Autodesk Inventor part; units mm, degrees
ref_plane "YZ Plane" through (0, 0, 0) normal (1, 0, 0) x (0, 1, 0)
ref_plane "XZ Plane" through (0, 0, 0) normal (0, 1, 0) x (-1, 0, 0)
ref_plane "XY Plane" through (0, 0, 0) normal (0, 0, 1) x (1, 0, 0)
sketch "Sketch1" plane through (0, 0, 0) normal (0, 1, 0) x (-1, 0, 0)
  line L0 (0, 0) -> (25.4, 0)
  line L1 (25.4, 0) -> (25.4, -180.34)
  line L2 (25.4, -180.34) -> (0, -180.34)
  line L3 (0, -180.34) -> (0, 0)
  dimension "d0" = 25.4
  dimension "d1" = 180.34
extrude "Plate1" add sketch "Sketch1" along normal blind 3.048
sketch "Sketch2" plane through (3.048, 6.096, -180.34) normal (1, 0, 0) x (0, 1, 0)
  line L0 (0, 180.34) -> (0, 0)
  line L1 (0, 0) -> (19.304, 0)
  line L2 (19.304, 0) -> (19.304, 180.34)
  line L3 (19.304, 180.34) -> (0, 180.34)
edge flange "Flange1" height 25.4 angle 90 thickness 3.048 bend radius 3.048 thickness toward (1, 0, 0) relief tear relief width 3.048 relief depth 1.524 edges at (0, 3.048, -90.17) wall of the first edge with corners at (3.048, 6.096, 0) (3.048, 6.096, -180.34) (3.048, 25.4, -180.34) (3.048, 25.4, 0)
bend "Bend1"
corner "Corner1"
sketch "Sketch3" plane through (0, 0, 0) normal (0, -1, 0) x (1, 0, 0)
  line L0 (-25.4, 0) -> (-25.4, -180.34)
  line L1 (-25.4, -180.34) -> (0, -180.34) construction
  line L2 (-12.7, -180.34) -> (-12.7, -150.2833) construction
  line L3 (-12.7, -150.2833) -> (-12.7, -120.2267) construction
  line L4 (-12.7, -120.2267) -> (-12.7, -90.17) construction
  line L5 (-12.7, -90.17) -> (-12.7, -60.1133) construction
  line L6 (-12.7, -60.1133) -> (-12.7, -30.0567) construction
  line L7 (-12.7, -30.0567) -> (-12.7, 0) construction
  line L8 (0, 0) -> (-25.4, 0) construction
  dimension "d13" = 12.7
hole "Hole1" at (-12.7, 0, -120.2267) at (-12.7, 0, -150.2833) at (-12.7, 0, -90.17) at (-12.7, 0, -60.1133) at (-12.7, 0, -30.0567) direction (0, 1, 0) diameter 3.5719 depth 3.048 tip angle 118
sketch "Sketch4" plane through (6.096, 25.4, 0) normal (1, 0, 0) x (0, 0, -1)
  line L0 (0, -12.7) -> (30.0567, -12.7) construction
  line L1 (30.0567, -12.7) -> (60.1133, -12.7) construction
  line L2 (60.1133, -12.7) -> (90.17, -12.7) construction
  line L3 (90.17, -12.7) -> (120.2267, -12.7) construction
  line L4 (120.2267, -12.7) -> (150.2833, -12.7) construction
  line L5 (150.2833, -12.7) -> (180.34, -12.7) construction
  line L6 (180.34, -25.4) -> (0, -25.4)
  line L7 (180.34, 0) -> (180.34, -19.304)
  line L8 (0, -19.304) -> (0, 0)
  dimension "d21" = 12.7
hole "Hole2" at (6.096, 12.7, -30.0567) at (6.096, 12.7, -60.1133) at (6.096, 12.7, -90.17) at (6.096, 12.7, -120.2267) at (6.096, 12.7, -150.2833) direction (-1, 0, 0) diameter 3.5719 depth 3.048 tip angle 118
equation "\"d0\" = cb_outer_diameter"
equation "\"d1\" = bh_length"
equation "\"d13\" = 0.5 * cb_outer_diameter"
equation "\"d14\" = rv_hole_diameter"
equation "\"d19\" = Thickness"
equation "\"d21\" = 0.5 * cb_outer_diameter"
equation "\"d22\" = rv_hole_diameter"
equation "\"d27\" = Thickness"
equation "\"d3\" = BendReliefWidth"
equation "\"d4\" = BendReliefDepth"
equation "\"d5\" = MinimumRemnant"
equation "\"d6\" = BendRadius"
equation "\"d9\" = BendRadius"
equation "\"d10\" = CornerReliefSize"
equation "\"d11\" = GapSize"
equation "\"d12\" = JacobiRadiusSize"
equation "\"BendRadius\" = Thickness"
equation "\"BendReliefWidth\" = Thickness"
equation "\"BendReliefDepth\" = 0.5 * Thickness"
equation "\"CornerReliefSize\" = 4 * Thickness"
equation "\"MinimumRemnant\" = 2 * Thickness"
equation "\"TransitionRadius\" = BendRadius"
equation "\"JacobiRadiusSize\" = BendRadius"
equation "\"GapSize\" = Thickness"
equation "\"bh_width\" = 87.63"
equation "\"bh_length\" = 180.34"
equation "\"bh_height\" = 25.4"
equation "\"bh_metal_width\" = 3.048"
equation "\"cpn_diameter\" = 69.85"
equation "\"cpn_length\" = 311.15"
equation "\"cmp_foot_seperation_long\" = 139.954"
equation "\"cmp_foot_seperation_short\" = 36.068"
equation "\"cmp_mounting_margins\" = 6.35"
equation "\"cmp_foot_bolt_diameter\" = 6.35"
equation "\"spd_fillet_size\" = 3.175"
equation "\"cb_outer_diameter\" = 25.4"
equation "\"cb_wall_thickness\" = 1.5875"
equation "\"cb_length\" = 508"
equation "\"pdb_mounting_holes_short\" = 104.394"
equation "\"cb_pdb_low_mount_offset\" = 25.4"
equation "\"pdb_mounting_holes_long\" = 182.2704"
equation "\"pdb_ziptie_hole_diameter\" = 5.334"
equation "\"d2\" = BendRadius"
equation "\"rv_hole_diameter\" = 3.57187"
properties part number "long_angle_bracket"
Could you check a few things on this model? Use its own coordinates, in mm. A direction names the side the tool comes from. Coordinates: 2 decimals unless noted, no trailing zeros. Order: outer loops, then holes, each group sorted by start corner. A loop starts at its lowest first (then second) coordinate and runs counter-clockwise, first axis right, second up. Notation, with made-up numbers: M 14,-10 L 40,-10 A23 cw 40,29 Z; hole C 70.25,44 d7. An arc over 180 degrees is marked long. Use a Markdown table: item, result. Add a question column.
Q1. I want a section at D-D on z = -53. List the corners of the cut face in (x, y) for me, then the cut area to 3 significant figures.
Q2. I want a section at C-C on z = -90.17. List the corners of the cut face in (x, y) for me.
Q3. I want a section at B-B on x = -12.7. List the corners of the cut face in (y, z) for me, then the cut area to 3 significant figures.
Q4. We'd pull the mould along X, two halves only. Please class faces 1 (the cylindrical face through (-12.779, 1.545, -88.386)), 2 (the cylindrical face through (4.358, 1.833, -91.432)), 3 (the cylindrical face through (4.551, 12.621, -88.386)), 4 (the cylindrical face through (-13.24, 1.55, -121.93)): pulls with the +X half, pulls with the -X half, needs draft (parallel to the pull), parting line crosses it, or undercut.
Q5. I want a section at A-A on y = 12.7. List the corners of the cut face in (x, z) for me.
Q6. If I drill on L1, parallel to Z at x = -12.7, y = 1; L2, parallel to X at y = 19.5, z = -40.5; L3, parallel to Y at x = -22.5, z = -90.5, over which ranges is the centre line in solid material (lowest first)?
Q7. Which directions (+Z, -Z, +X, -X, +Y, -Y) give clear straight access to the entire face, cutting with the end or side of a thin tool? Please do faces 5 (the flat face through (-15, 3.048, -89)), 6 (the cylindrical face through (-13.236, 1.545, -61.817)).
Q8. I'm going to push flat-ended pins straight in: pin 1 (6 mm diameter, centred on x = -17, z = -81.5, fed in from +Y); pin 2 (8 mm diameter, centred on y = 17, z = -22.5, fed in from -X). Where does each tip first touch, or does it pass through?
Checked values:
| question | item | result |
|---|---|---|
| 1 | outline | M -25.4,0 L 0,0 A6.1 ccw 6.1,6.1 L 6.1,25.4 L 3.05,25.4 L 3.05,6.1 A3.05 cw 0,3.05 L -25.4,3.05 Z |
| 1 | area | 158 mm² |
| 2 | outline | M -25.4,0 L -14.49,0 L -14.49,3.05 L -25.4,3.05 Z; M -10.91,0 L 0,0 A6.1 ccw 6.1,6.1 L 6.1,10.91 L 3.05,10.91 L 3.05,6.1 A3.05 cw 0,3.05 L -10.91,3.05 Z; M 3.05,14.49 L 6.1,14.49 L 6.1,25.4 L 3.05,25.4 Z |
| 3 | outline | M 0,-180.34 L 3.05,-180.34 L 3.05,-152.07 L 0,-152.07 Z; M 0,-148.5 L 3.05,-148.5 L 3.05,-122.01 L 0,-122.01 Z; M 0,-118.44 L 3.05,-118.44 L 3.05,-91.96 L 0,-91.96 Z; M 0,-88.38 L 3.05,-88.38 L 3.05,-61.9 L 0,-61.9 Z; M 0,-58.33 L 3.05,-58.33 L 3.05,-31.84 L 0,-31.84 Z; M 0,-28.27 L 3.05,-28.27 L 3.05,0 L 0,0 Z |
| 3 | area | 495 mm² |
| 4 | face 1 | undercut |
| 4 | face 2 | pulls with the +X half |
| 4 | face 3 | needs draft |
| 4 | face 4 | undercut |
| 5 | outline | M 3.05,-180.34 L 6.1,-180.34 L 6.1,-152.07 L 3.05,-152.07 Z; M 3.05,-148.5 L 6.1,-148.5 L 6.1,-122.01 L 3.05,-122.01 Z; M 3.05,-118.44 L 6.1,-118.44 L 6.1,-91.96 L 3.05,-91.96 Z; M 3.05,-88.38 L 6.1,-88.38 L 6.1,-61.9 L 3.05,-61.9 Z; M 3.05,-58.33 L 6.1,-58.33 L 6.1,-31.84 L 3.05,-31.84 Z; M 3.05,-28.27 L 6.1,-28.27 L 6.1,0 L 3.05,0 Z |
| 6 | L1 | -180.34 to -152.07, -148.5 to -122.01, -118.44 to -91.96, -88.38 to -61.9, -58.33 to -31.84, -28.27 to 0 |
| 6 | L2 | 3.05 to 6.1 |
| 6 | L3 | 0 to 3.05 |
| 7 | face 5 | +Z, -Z, -X, +Y |
| 7 | face 6 | +Y, -Y |
| 8 | pin 1 | y = 3.05 |
| 8 | pin 2 | x = 3.05 |
